```python
from build123d import *

# Parameters (mm, degrees)
SKETCH1_R           = 3.737759178
SKETCH1_W           = 50.524481644
SKETCH1_H           = 6
BOSS_EXTRUDE1_DEPTH = 2.18


with BuildPart() as part:
    # Sketch1 → Boss-Extrude1 (new body)
    # profile 1 of 7: a face of its own
    with BuildSketch(Plane.XY):
        with Locations((-29, 11.5)):
            Circle(SKETCH1_R)
        with BuildLine():
            ThreePointArc((-29, 10.15), (-27.65, 11.5), (-29, 12.85))
            ThreePointArc((-29, 12.85), (-30.35, 11.5), (-29, 10.15))
        make_face(mode=Mode.SUBTRACT)
    # profile 2 of 7: a face of its own
    with BuildSketch(Plane.XY):
        with BuildLine():
            Line((-25.262240822, 3), (-25.262240822, 11.5))
            ThreePointArc((-25.262240822, 11.5), (-29, 7.762240822), (-32.737759178, 11.5))
            Line((-32.737759178, 11.5), (-32.737759178, -11.5))
            ThreePointArc((-32.737759178, -11.5), (-29, -7.762240822), (-25.262240822, -11.5))
            Line((-25.262240822, -11.5), (-25.262240822, -3))
            Line((-25.262240822, -3), (-25.262240822, 3))
        make_face()
    # profile 3 of 7: a face of its own
    with BuildSketch(Plane.XY):
        with Locations((-29, -11.5)):
            Circle(SKETCH1_R)
        with BuildLine():
            ThreePointArc((-29, -10.15), (-30.35, -11.5), (-29, -12.85))
            ThreePointArc((-29, -12.85), (-27.65, -11.5), (-29, -10.15))
        make_face(mode=Mode.SUBTRACT)
    # profile 4 of 7: a face of its own
    with BuildSketch(Plane.XY):
        Rectangle(SKETCH1_W, SKETCH1_H)
    # profile 5 of 7: a face of its own
    with BuildSketch(Plane.XY):
        with BuildLine():
            Line((25.262240822, 11.5), (25.262240822, 3))
            Line((25.262240822, 3), (25.262240822, -3))
            Line((25.262240822, -3), (25.262240822, -11.5))
            ThreePointArc((25.262240822, -11.5), (29, -7.762240822), (32.737759178, -11.5))
            Line((32.737759178, -11.5), (32.737759178, 11.5))
            ThreePointArc((32.737759178, 11.5), (29, 7.762240822), (25.262240822, 11.5))
        make_face()
    # profile 6 of 7: a face of its own
    with BuildSketch(Plane.XY):
        with Locations((29, 11.5)):
            Circle(SKETCH1_R)
        with BuildLine():
            ThreePointArc((29, 10.15), (30.35, 11.5), (29, 12.85))
            ThreePointArc((29, 12.85), (27.65, 11.5), (29, 10.15))
        make_face(mode=Mode.SUBTRACT)
    # profile 7 of 7: a face of its own
    with BuildSketch(Plane.XY):
        with Locations((29, -11.5)):
            Circle(SKETCH1_R)
        with BuildLine():
            ThreePointArc((29, -12.85), (30.35, -11.5), (29, -10.15))
            ThreePointArc((29, -10.15), (27.65, -11.5), (29, -12.85))
        make_face(mode=Mode.SUBTRACT)
    extrude(amount=BOSS_EXTRUDE1_DEPTH)


solid = part.part
```
The model under review builds one solid part; all positions refer to its coordinate system, in mm. A direction names the side the tool comes from. Give positions to 0.01 mm unless a question says otherwise; leave off trailing zeros. Write each loop counter-clockwise with the first axis right and the second up, starting at its lowest first coordinate (ties: lowest second). Pieces come first, ordered by that corner, then holes. Notation, with made-up numbers: (48, 10) -> (52, 10) arc R18 ccw to (52, 39) -> close; hole circle Ø9 at (82, -29). An arc over 180 degrees is marked (long way). Answer in a Markdown table with one row per item.
1) Add section A-A on y = -8.5. State the section outline as (x, z) points.
Worked answers:
| item | result |
|---|---|
| outline | (-32.74, 0) -> (-25.26, 0) -> (-25.26, 2.18) -> (-32.74, 2.18) -> close; (25.26, 0) -> (32.74, 0) -> (32.74, 2.18) -> (25.26, 2.18) -> close |
2) For L1, parallel to Y at x = 29, z = 1.7; L2, parallel to X at y = -11.5, z = 1.4; L3, parallel to X at y = -3.5, z = 0.95, list the stretches that pass through material, from the lowest coordinate up. Write a range as [from, to].
Worked answers:
| item | result |
|---|---|
| L1 | [-15.24, -12.85], [-10.15, 10.15], [12.85, 15.24] |
| L2 | [-32.74, -30.35], [-27.65, -25.26], [25.26, 27.65], [30.35, 32.74] |
| L3 | [-32.74, -25.26], [25.26, 32.74] |
3) Mouldability with a two-part tool opening along Y and no side actions: class faces 1 (the cylindrical face through (30.2, -10.88, 1.07)), 2 (the flat face through (32.738, 0, 1)), 3 (the cylindrical face through (30.2, 12.12, 1.07)), 4 (the cylindrical face through (29.082, 15.237, 1.075)) as +Y half, -Y half, draft (parallel to the pull), parting line (faces both ways), or undercut.
Worked answers:
| item | result |
|---|---|
| face 1 | undercut |
| face 2 | draft |
| face 3 | undercut |
| face 4 | +Y half |
4) Clearance check with a flat-ended pin moving along its axis: P1, Ø6, axis at x = -22, y = -7.5, coming from the -Z side. State where the tip first meets the part, or that it passes through.
Worked answers:
| item | result |
|---|---|
| P1 | through |
5) Add section B-B on z = 0.6. State the section outline as (x, y) points, plus the area to 3 significant figures.
Worked answers:
| item | result |
|---|---|
| outline | (-32.74, -11.5) arc R3.74 ccw to (-25.26, -11.5) -> (-25.26, -3) -> (25.26, -3) -> (25.26, -11.5) arc R3.74 ccw to (32.74, -11.5) -> (32.74, 11.5) arc R3.74 ccw to (25.26, 11.5) -> (25.26, 3) -> (-25.26, 3) -> (-25.26, 11.5) arc R3.74 ccw to (-32.74, 11.5) -> close; hole circle Ø2.7 at (-29, -11.5); hole circle Ø2.7 at (-29, 11.5); hole circle Ø2.7 at (29, -11.5); hole circle Ø2.7 at (29, 11.5) |
| area | 712 mm² |
6) Add section C-C on x = 29. State the section outline as (y, z) points, plus the area to 3 significant figures.
Worked answers:
| item | result |
|---|---|
| outline | (-15.24, 0) -> (-12.85, 0) -> (-12.85, 2.18) -> (-15.24, 2.18) -> close; (-10.15, 0) -> (10.15, 0) -> (10.15, 2.18) -> (-10.15, 2.18) -> close; (12.85, 0) -> (15.24, 0) -> (15.24, 2.18) -> (12.85, 2.18) -> close |
| area | 54.7 mm² |
7) Tool access review of faces 5 (the flat face through (25.262, -7, 1)), 6 (the flat face through (-25.262, 7, 1)), 7 (the flat face through (0, 1, 2.18)): name each direction out of +Z, -Z, +X, -X, +Y, -Y from which nothing blocks a thin tool from reaching the whole face with its end or side.
Worked answers:
| item | result |
|---|---|
| face 5 | +Z, -Z, -Y |
| face 6 | +Z, -Z, +Y |
| face 7 | +Z, +X, -X, +Y, -Y |
